Autodesk Inventor part; units mm, degrees
ref_plane "YZ Plane" through (0, 0, 0) normal (1, 0, 0) x (0, 1, 0)
ref_plane "XZ Plane" through (0, 0, 0) normal (0, 1, 0) x (-1, 0, 0)
ref_plane "XY Plane" through (0, 0, 0) normal (0, 0, 1) x (1, 0, 0)
sketch "Sketch1" plane through (0, 0, 0) normal (0, 0, 1) x (1, 0, 0)
  line L0 (0, 0) -> (-254, 0)
  line L1 (-254, 406.4) -> (0, 406.4)
  line L2 (0, 406.4) -> (0, 0)
  line L3 (-254, 0) -> (-254, 155.9052)
  line L4 (-285.75, 187.6552) -> (-355.6, 187.6552)
  circle A0 centre (-95.25, 190.5) radius 38.1
  arc A1 (-254, 155.9052) -> (-285.75, 187.6552) centre (-285.75, 155.9052) ccw
  circle A2 centre (-330.2, 463.55) radius 19.05
  line L5 (-515.6961, 0) -> (516.0768, 0)
  line L6 (-368.3, 304.8) -> (-355.6, 187.6552)
  circle A3 centre (-228.6, 355.6) radius 19.05
  circle A4 centre (279.7806, 579.9282) radius 88.9
  circle A5 centre (-152.4, 276.86) radius 19.05
  line L7 (-336.55, 187.6552) -> (-368.3, 304.8)
  point P0 (-254, 187.6552)
  dimension "d0" = 406.4
  dimension "d4" = 158.75
  dimension "d5" = 190.5
  dimension "d6" = 76.2
  dimension "d13" = 31.75
  dimension "d14" = 463.55
  dimension "d20" = 330.2
  dimension "d54" = 101.6
  dimension "d59" = 254
  dimension "d61" = 304.8
  dimension "d62" = 187.6552
  dimension "d63" = 12.7
  dimension "d76" = 38.1
  dimension "d87" = 228.6
  dimension "d88" = 355.6
  dimension "d89" = 38.1
  dimension "d90" = 177.8
  dimension "d91" = 38.1
  dimension "d92" = 276.86
  dimension "d93" = 152.4
  dimension "d94" = 82.55
sketch "Sketch5" plane through (0, 0, 0) normal (0, 0, 1) x (1, 0, 0)
  line L0 (-346.559, 517.9919) -> (-91.3724, 246.8562)
  line L1 (-91.3724, 246.8562) -> (-49.3064, 146.7099)
  line L2 (-49.3064, 146.7099) -> (-96.1423, 127.0367)
  line L3 (-96.1423, 127.0367) -> (-134.6544, 218.7223)
  line L4 (-134.6544, 218.7223) -> (-383.5128, 483.1343)
  line L5 (-383.5128, 483.1343) -> (-346.5202, 517.9508)
  point P0 (0, 0)
  point P1 (-95.25, 190.5)
  point P2 (-152.4, 276.86)
  point P3 (-228.6, 355.6)
  point P4 (-330.2, 463.55)
  dimension "d107" = 50.8
  dimension "d108" = 50.8
  dimension "d109" = 25.4
  dimension "d110" = 25.4
  dimension "d111" = 25.4
  dimension "d113" = 50.8
extrude "Extrusion4" add sketch "Sketch5" along normal blind 25.4
hole "Hole1" at (-95.25, 190.5, 0) at (-152.4, 276.86, 0) at (-228.6, 355.6, 0) at (-330.2, 463.55, 0) direction (0, 0, 1) diameter 22.225 end through all
sketch "Sketch6" plane through (0, 0, 25.4) normal (0, 0, 1) x (1, 0, 0)
  line L0 (-108.2166, 155.7818) -> (-61.3806, 175.455)
  line L1 (-49.3064, 146.7099) -> (-91.3724, 246.8562)
  line L2 (-61.3806, 175.455) -> (-49.3064, 146.7099)
  line L3 (-134.6544, 218.7223) -> (-96.1423, 127.0367)
  line L4 (-49.3064, 146.7099) -> (-96.1423, 127.0367)
  line L5 (-96.1423, 127.0367) -> (-108.2166, 155.7818)
  circle A0 centre (-95.25, 190.5) radius 11.1125
  point P0 (0, 0)
  dimension "d123" = 26.9875
extrude "Extrusion5" cut sketch "Sketch6" against normal blind 25.4 contours L0 L1 L4 L3
shell "Shell1" thickness 1.5875 removed faces 2 at (-92.6046, 162.3395, 8.4667) at (-358.8511, 506.3453, 8.4667)
sketch "Sketch7" plane through (-383.5128, 483.1343, 25.4) normal (-0.6854, 0.7282, 0) x (0.7282, 0.6854, 0)
  line L0 (49.2125, 1.5875) -> (1.5875, 1.5875)
  line L1 (1.5875, 1.5875) -> (1.5875, 23.8125)
  line L2 (49.2125, 1.5875) -> (1.5875, 1.5875)
  line L3 (1.5875, 1.5875) -> (1.5875, 23.8125)
  line L4 (1.5875, 23.8125) -> (49.2125, 23.8125)
  line L5 (49.2125, 23.8125) -> (49.2125, 1.5875)
  point P0 (-51.8492, 25.4)
extrude "Extrusion6" cut sketch "Sketch7" against normal blind 330.2
sketch "Sketch8" plane through (-108.2166, 155.7818, 0) normal (0.3873, -0.922, 0) x (0.922, 0.3873, 0)
  line L0 (49.2125, 1.5875) -> (49.2125, 23.8125)
  line L1 (49.2125, 1.5875) -> (1.5875, 1.5875)
  line L2 (1.5875, 1.5875) -> (1.5875, 23.8125)
  line L3 (1.5875, 23.8125) -> (49.2125, 23.8125)
  line L4 (49.2125, 23.8125) -> (49.2125, 1.5875)
  point P0 (39.4428, 0)
extrude "Extrusion7" cut sketch "Sketch8" against normal blind 76.2
sketch "Sketch9" plane through (0, 0, 25.4) normal (0, 0, 1) x (1, 0, 0)
  line L0 (-382.3568, 484.2223) -> (-133.3019, 219.6015)
  line L1 (-91.3724, 246.8562) -> (-346.5202, 517.9508)
  line L2 (-61.3806, 175.455) -> (-91.3724, 246.8562)
  line L3 (-91.3724, 246.8562) -> (-61.3806, 175.455)
  line L4 (-134.6544, 218.7223) -> (-108.2166, 155.7818)
  line L5 (-61.3806, 175.455) -> (-108.2166, 155.7818)
  line L6 (-108.2166, 155.7818) -> (-134.6544, 218.7223)
  line L7 (-383.5128, 483.1343) -> (-134.6544, 218.7223)
  line L8 (-91.3724, 246.8562) -> (-134.6544, 218.7223)
  line L9 (-91.3724, 246.8562) -> (-141.3682, 225.8557)
  line L10 (-91.3724, 246.8562) -> (-130.8608, 209.6907)
  line L11 (-346.5202, 517.9508) -> (-383.5128, 483.1343)
  point P0 (0, 0)
sketch "Sketch10" plane through (0, 0, 25.4) normal (0, 0, 1) x (1, 0, 0)
  circle A0 centre (-948.4671, 602.0735) radius 85.2109
  circle A1 centre (-704.3018, 697.4759) radius 79.8897
  point P0 (0, 0)
sketch "Sketch11" plane through (0, 0, 0) normal (0, 0, -1) x (-1, 0, 0)
  line L0 (61.3806, 175.455) -> (91.3724, 246.8562)
  line L1 (91.3724, 246.8562) -> (141.3682, 225.8557)
  line L2 (383.5128, 483.1343) -> (134.6544, 218.7223)
  line L3 (61.3806, 175.455) -> (108.2166, 155.7818)
  line L4 (134.6544, 218.7223) -> (108.2166, 155.7818)
  line L5 (91.3724, 246.8562) -> (134.6544, 218.7223)
  line L6 (91.3724, 246.8562) -> (346.5202, 517.9508)
  line L7 (91.3724, 246.8562) -> (130.8607, 209.6906)
  point P0 (0, 0)
  dimension "d131" = 10.24
properties part number "RollerIntakePrototype 2.0 3 WHEELS"
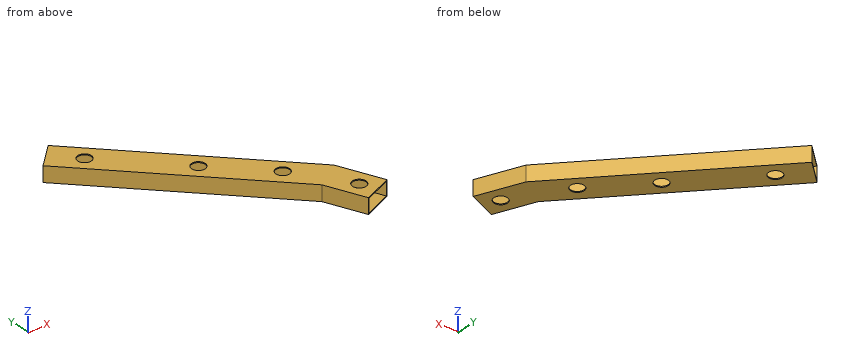
Input: part model. Units: mm. Frame: model coordinates. Coordinates: 2 decimals unless noted, no trailing zeros. Write each loop counter-clockwise with the first axis right and the second up, starting at its lowest first coordinate (ties: lowest second). Pieces come first, ordered by that corner, then holes. Notation, with made-up numbers: (9.25, 89.5) - (21.25, 89.5) arc R14 ccw to (21.25, 94.5) - close; hole circle Ø10 at (89.5, -14). An arc over 180 degrees is marked (long way). Put each result on its own line as item: value. Start each with the question number.
1) Contact query for flat-ended pins moving along their axis: pin 1 (18 mm diameter, centred on x = -95.25, y = 190.5, fed in from -Z); pin 2 (2 mm diameter, centred on y = 315.5, z = 17, fed in from +X); pin 3 (3 mm diameter, centred on y = 330, z = 4.5, fed in from -X); pin 4 (12 mm diameter, centred on x = -136.5, z = 5, fed in from -Y). Output: stop coordinate, or through.
2) Ray query, L1, parallel to Y at x = -152.4, z = 24.5; L2, parallel to X at y = 178.5, z = 11.5; L3, parallel to Y at x = -330.2, z = 25. Return the intervals inside material, ascending.
3) Cut plane B-B (x = -152.4). Return the cut outline in (y, z).
4) Cut plane D-D (z = 6.75). Return the cut outline in (x, y) (3 decimals).
5) Cut plane C-C (x = -210.5). Return the cut outline in (y, z).
6) Cut plane A-A (y = 190.5). Return the cut outline in (x, z), plus the area to 3 significant figures.
Resolved:
1. pin 1: passes through
1. pin 2: stops at x = -155.04
1. pin 3: stops at x = -240.8
1. pin 4: stops at y = 208.83
2. L1: y = 237.58 to 265.75, 287.97 to 311.7
2. L2: x = -117.76 to -116.04, -64.38 to -62.66
2. L3: y = 426.49 to 452.44, 474.66 to 500.61
3. outline: (237.58, 0) - (265.75, 0) - (265.75, 1.59) - (239.89, 1.59) - (239.89, 23.81) - (265.75, 23.81) - (265.75, 25.4) - (237.58, 25.4) - close; (287.97, 0) - (311.7, 0) - (311.7, 25.4) - (287.97, 25.4) - (287.97, 23.81) - (309.39, 23.81) - (309.39, 1.59) - (287.97, 1.59) - close
4. outline: (-383.513, 483.134) - (-134.654, 218.722) - (-108.217, 155.782) - (-106.753, 156.397) - (-133.304, 219.604) - (-382.357, 484.222) - close; (-347.676, 516.863) - (-121.362, 276.416) - (-121.368, 276.411) - (-92.725, 245.977) - (-62.844, 174.84) - (-61.381, 175.455) - (-91.372, 246.856) - (-346.52, 517.951) - close
5. outline: (299.31, 0) - (373.43, 0) - (373.43, 25.4) - (299.31, 25.4) - close; hole (301.62, 1.59) - (371.12, 1.59) - (371.12, 23.81) - (301.62, 23.81) - close
6. outline: (-122.8, 0) - (-106.36, 0) - (-106.36, 1.59) - (-121.08, 1.59) - (-121.08, 23.81) - (-106.36, 23.81) - (-106.36, 25.4) - (-122.8, 25.4) - close; (-84.14, 0) - (-67.7, 0) - (-67.7, 25.4) - (-84.14, 25.4) - (-84.14, 23.81) - (-69.42, 23.81) - (-69.42, 1.59) - (-84.14, 1.59) - close
6. area: 181 mm2
